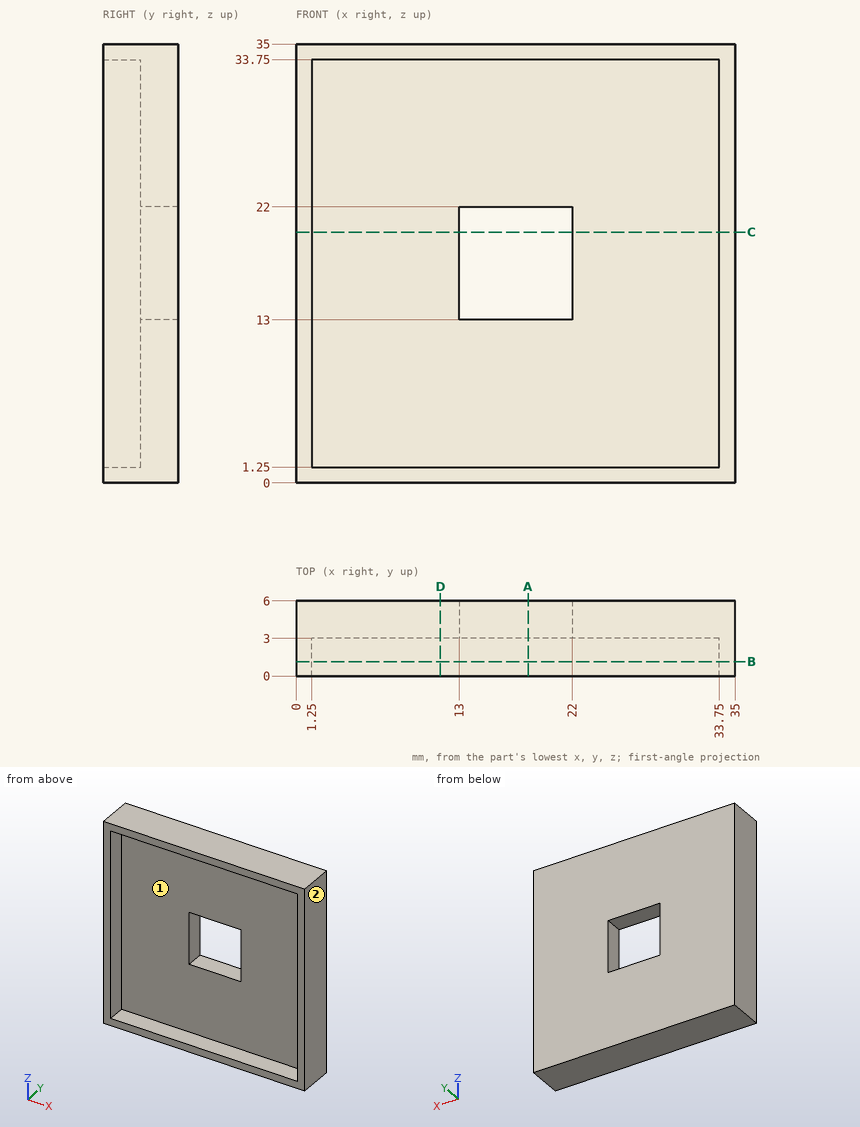
Verification items for this drawing (mm, ordinates from the low corner). A direction names the side the tool comes from. Coordinates: 2 decimals unless noted, no trailing zeros. Loops run counter-clockwise (first coordinate to the right, second up) from the corner with the lowest first, then second, coordinate; pieces in that order, holes last.
Item 1: Thickness scan on line 1 (X direction, y = 1.5, z = 24.5); line 2 (Z direction, x = 15, y = 5.7). Record the ranges inside material, lowest first.
Item 2: Sectioned sample at A-A, the plane x = 18.5. Record the boundary of the cut face in (y, z).
Item 3: Sectioned sample at D-D, the plane x = 11.5. Record the boundary of the cut face in (y, z).
Item 4: Access from +Z, -Z, +X, -X, +Y, -Y to the whole of each face (thin tool, end or side, straight path). Record for the marked faces 1 and 2.
Item 5: Go/stop test with a flat-tipped pin: pin 1 Ø1.5 at (x, z) = (31.5, 4) entering from -Y. Record where the tip stops, or that it passes through.
Item 6: Sectioned sample at C-C, the plane z = 20. Record the boundary of the cut face in (x, y), then the cut area to 3 significant figures.
Item 7: Sectioned sample at B-B, the plane y = 1.15. Record the boundary of the cut face in (x, z), then the cut area to 3 significant figures.
Check result:
1. line 1: x = 0 to 1.25, 33.75 to 35
1. line 2: z = 0 to 13, 22 to 35
2. outline: (0, 0) - (6, 0) - (6, 13) - (3, 13) - (3, 1.25) - (0, 1.25) - close; (0, 33.75) - (3, 33.75) - (3, 22) - (6, 22) - (6, 35) - (0, 35) - close
3. outline: (0, 0) - (6, 0) - (6, 35) - (0, 35) - (0, 33.75) - (3, 33.75) - (3, 1.25) - (0, 1.25) - close
4. face 1: -Y
4. face 2: +Z, -Z, +X, +Y, -Y
5. pin 1: stops at y = 3
6. outline: (0, 0) - (1.25, 0) - (1.25, 3) - (13, 3) - (13, 6) - (0, 6) - close; (22, 3) - (33.75, 3) - (33.75, 0) - (35, 0) - (35, 6) - (22, 6) - close
6. area: 85.5 mm2
7. outline: (0, 0) - (35, 0) - (35, 35) - (0, 35) - close; hole (1.25, 1.25) - (33.75, 1.25) - (33.75, 33.75) - (1.25, 33.75) - close
7. area: 169 mm2
